Verification items for this drawing (mm, ordinates from the low corner). A direction names the side the tool comes from. Give positions to 0.01 mm unless a question says otherwise; leave off trailing zeros. Loops run counter-clockwise (first coordinate to the right, second up) from the corner with the lowest first, then second, coordinate; pieces in that order, holes last. Notation, with made-up numbers: (10, 21) -> (44, 21) arc R22 cw to (44, 38) -> close; hole circle Ø1 at (12, 58.5). An arc over 180 degrees is marked (long way). Answer as a JSON object with one key per item and string values.
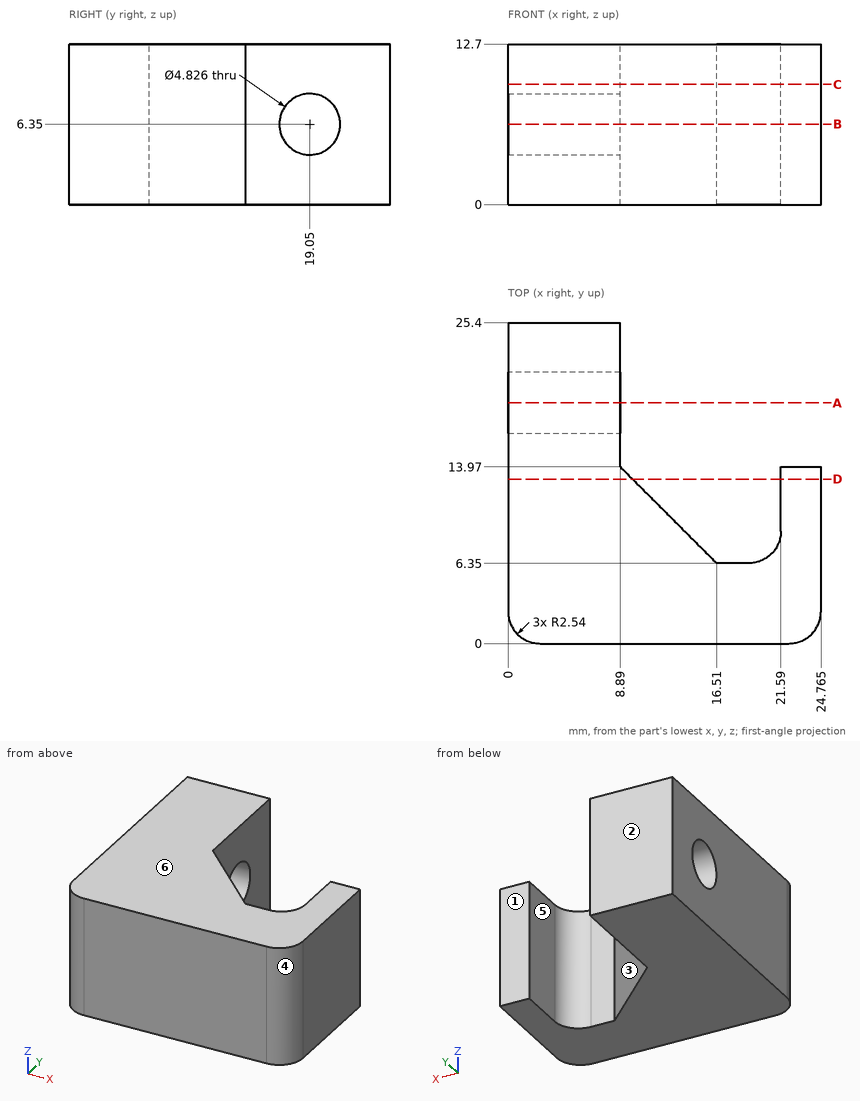
1) Section check A-A on y = 19.05. Record the cut outline in (x, z), plus the area to 3 significant figures.
Geometry check:
{"outline": "(0, 0) -> (8.89, 0) -> (8.89, 3.94) -> (0, 3.94) -> close; (0, 8.76) -> (8.89, 8.76) -> (8.89, 12.7) -> (0, 12.7) -> close", "area": "70.0 mm2"}
2) Depth check by flat-ended pin: P1, Ø5.5, axis at y = 19.5, z = 9.5, coming from the +X side; P2, Ø1, axis at x = 23.5, z = 8.5, coming from the +Y side; P3, Ø2, axis at x = 18, z = 6.5, coming from the +Y side. Enter the tip coordinate at first touch or a pass-through.
Geometry check:
{"P1": "stops at x = 8.89", "P2": "stops at y = 13.97", "P3": "stops at y = 6.35"}
3) Tool access check on the marked faces 1, 2 and 3. Record the directions out of +Z, -Z, +X, -X, +Y, -Y that give a thin tool (end or side, any length) a straight path to the whole face; none if there is none.
Geometry check:
{"face 1": "+Z, -Z, +X, +Y", "face 2": "+Z, -Z, +X, -X, +Y", "face 3": "+Z, -Z, +Y"}
4) Material ranges on line 1 along Z through (x, y) = (4, 19.05); line 2 along X through (y, z) = (18.5, 3.5); line 3 along X through (y, z) = (10.75, 12) (3 decimals), recorded low to high. Write a range as from..to.
Geometry check:
{"line 1": "z = 0..3.94, 8.76..12.7", "line 2": "x = 0..8.89", "line 3": "x = 0..12.11, 21.59..24.765"}
5) Section check D-D on y = 13. Record the cut outline in (x, z) (3 decimals), plus the area to 3 significant figures.
Geometry check:
{"outline": "(0, 0) -> (9.86, 0) -> (9.86, 12.7) -> (0, 12.7) -> close; (21.59, 0) -> (24.765, 0) -> (24.765, 12.7) -> (21.59, 12.7) -> close", "area": "166 mm2"}
6) Section check B-B on z = 6.35. Record the cut outline in (x, y) (3 decimals).
Geometry check:
{"outline": "(0, 2.54) arc R2.54 ccw to (2.54, 0) -> (22.225, 0) arc R2.54 ccw to (24.765, 2.54) -> (24.765, 13.97) -> (21.59, 13.97) -> (21.59, 8.89) arc R2.54 cw to (19.05, 6.35) -> (16.51, 6.35) -> (8.89, 13.97) -> (8.89, 16.637) -> (0, 16.637) -> close; (0, 21.463) -> (8.89, 21.463) -> (8.89, 25.4) -> (0, 25.4) -> close"}
7) Section check C-C on z = 9.5. Record the cut outline in (x, y) (3 decimals).
Geometry check:
{"outline": "(0, 2.54) arc R2.54 ccw to (2.54, 0) -> (22.225, 0) arc R2.54 ccw to (24.765, 2.54) -> (24.765, 13.97) -> (21.59, 13.97) -> (21.59, 8.89) arc R2.54 cw to (19.05, 6.35) -> (16.51, 6.35) -> (8.89, 13.97) -> (8.89, 25.4) -> (0, 25.4) -> close"}
8) Draft check along X on the marked faces 4, 5 and 6. Enter one of: pulls with the +X half, pulls with the -X half, needs draft (parallel to the pull), parting line crosses it, or undercut.
Geometry check:
{"face 4": "pulls with the +X half", "face 5": "undercut", "face 6": "needs draft"}
